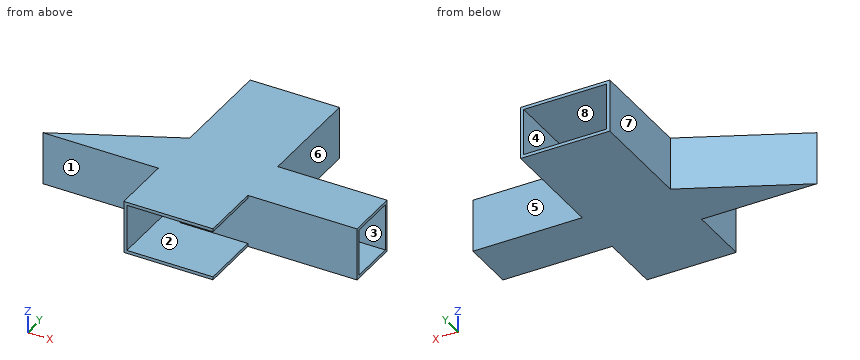
from build123d import *

# Parameters (mm, degrees)
ESQUISSE1_W             = 145
ESQUISSE1_H             = 86
ESQUISSE1_W_2           = 135
ESQUISSE1_H_2           = 76
BOSS_EXTRU_1_DEPTH      = 258
ESQUISSE2_W             = 145
ESQUISSE2_H             = 86
BOSS_EXTRU_2_DEPTH      = 5
ESQUISSE3_W             = 30
ESQUISSE3_H             = 76
ENL_V_MAT_EXTRU_1_DEPTH = 5
ESQUISSE5_W             = 5
ESQUISSE5_H             = 86
BOSS_EXTRU_3_DEPTH      = 100
BOSS_EXTRU_6_DEPTH      = 86
ESQUISSE10_W            = 86
ESQUISSE10_H            = 86
ESQUISSE10_W_2          = 76
ESQUISSE10_H_2          = 76
BOSS_EXTRU_7_DEPTH      = 177.5
ESQUISSE11_W            = 76
ESQUISSE11_H            = 76
ENL_V_MAT_EXTRU_2_DEPTH = 10
ESQUISSE12_W            = 140
ESQUISSE12_H            = 5
BOSS_EXTRU_8_DEPTH      = 100


with BuildPart() as part:
    # Esquisse1 → Boss.-Extru.1 (new body)
    with BuildSketch(Plane(origin=(0, 0, 0), x_dir=(1, 0, 0), z_dir=(0, 1, 0))):
        with Locations((34.799005462, -27.04875873)):
            Rectangle(ESQUISSE1_W, ESQUISSE1_H)
        with Locations((34.799005462, -27.04875873)):
            Rectangle(ESQUISSE1_W_2, ESQUISSE1_H_2, mode=Mode.SUBTRACT)
    extrude(amount=BOSS_EXTRU_1_DEPTH)

    # Esquisse2 → Boss.-Extru.2 (add)
    with BuildSketch(Plane.XZ):
        with Locations((34.799005462, 27.04875873)):
            Rectangle(ESQUISSE2_W, ESQUISSE2_H)
    extrude(amount=BOSS_EXTRU_2_DEPTH)

    # Esquisse3 → Enlèv. mat.-Extru.1 (cut)
    with BuildSketch(Plane.XZ.offset(5)):
        with Locations((-17.700994538, 27.04875873)):
            Rectangle(ESQUISSE3_W, ESQUISSE3_H)
    extrude(amount=-ENL_V_MAT_EXTRU_1_DEPTH, mode=Mode.SUBTRACT)

    # Esquisse5 → Boss.-Extru.3 (add)
    with BuildSketch(Plane.XZ.offset(5)):
        with Locations((-35.200994538, 27.04875873)):
            Rectangle(ESQUISSE5_W, ESQUISSE5_H)
    extrude(amount=BOSS_EXTRU_3_DEPTH)

    # Esquisse9 → Boss.-Extru.6 (add)
    with BuildSketch(Plane.XY.offset(70.04875873)):
        Polygon((-37.700994538, -5.700514768), (-37.700994538, 84.299485232), (-225.200994538, -5.700514768), align=None)
    extrude(amount=-BOSS_EXTRU_6_DEPTH)

    # Esquisse10 → Boss.-Extru.7 (add)
    with BuildSketch(Plane(origin=(107.299005462, 0, 0), x_dir=(0, 0, -1), z_dir=(1, 0, 0))):
        with Locations((-27.04875873, 38)):
            Rectangle(ESQUISSE10_W, ESQUISSE10_H)
        with Locations((-27.04875873, 38)):
            Rectangle(ESQUISSE10_W_2, ESQUISSE10_H_2, mode=Mode.SUBTRACT)
    extrude(amount=BOSS_EXTRU_7_DEPTH)

    # Esquisse11 → Enlèv. mat.-Extru.2 (cut)
    with BuildSketch(Plane(origin=(107.299005462, 0, 0), x_dir=(0, 0, -1), z_dir=(1, 0, 0))):
        with Locations((-27.04875873, 38)):
            Rectangle(ESQUISSE11_W, ESQUISSE11_H)
    extrude(amount=-ENL_V_MAT_EXTRU_2_DEPTH, mode=Mode.SUBTRACT)

    # Esquisse12 → Boss.-Extru.8 (add)
    with BuildSketch(Plane.XZ.offset(5)):
        with Locations((37.299005462, 67.54875873)):
            Rectangle(ESQUISSE12_W, ESQUISSE12_H)
        with Locations((37.299005462, -13.45124127)):
            Rectangle(ESQUISSE12_W, ESQUISSE12_H)
    extrude(amount=BOSS_EXTRU_8_DEPTH)


solid = part.part
Verification items for the finished model (mm, model axes). Face numbers are marked on the shaded views. A direction names the side the tool comes from. Give positions to 0.01 mm unless a question says otherwise; leave off trailing zeros. Loops run counter-clockwise (first coordinate to the right, second up) from the corner with the lowest first, then second, coordinate; pieces in that order, holes last.
1) Thickness scan on line 1 along X through (y, z) = (158.5, 45); line 2 along Z through (x, y) = (-25.5, 102.5); line 3 along Y through (x, z) = (260, 45.5). Record the ranges inside material, lowest first.
2) Depth check by flat-ended pin: pin 1 Ø4 at (y, z) = (-49.5, 45) entering from -X; pin 2 Ø6 at (x, z) = (72, 46) entering from +Y; pin 3 Ø1.5 at (y, z) = (-47.5, -13) entering from +X. Enter the tip coordinate at first touch or a pass-through.
3) Sectioned sample at C-C, the plane y = -72.5. Enter the section's corners in (x, z).
4) Sectioned sample at B-B, the plane z = 5. Enter the section's corners in (x, y), then the cut area to 3 significant figures.
5) Sectioned sample at A-A, the plane x = 133. Enter the section's corners in (y, z), then the cut area to 3 significant figures.
6) Draft check along X on the marked faces 6, 7 and 8. Enter one of: pulls with the +X half, pulls with the -X half, needs draft (parallel to the pull), parting line crosses it, or undercut.
7) Set-up check for the marked faces 1, 2, 3, 4 and 5: record each of +Z, -Z, +X, -X, +Y, -Y from which the full face is reachable in a straight line by a thin tool's end or side.
8) Sectioned sample at D-D, the plane x = 59. Enter the section's corners in (y, z), then the cut area to 3 significant figures.
Answers:
1. line 1: x = -37.7 to -32.7, 102.3 to 107.3
1. line 2: z = -15.95 to -10.95, 65.05 to 70.05
1. line 3: y = -5 to 0, 76 to 81
2. pin 1: stops at x = -37.7
2. pin 2: stops at y = 0
2. pin 3: stops at x = 107.3
3. outline: (-37.7, -15.95) - (107.3, -15.95) - (107.3, -10.95) - (-32.7, -10.95) - (-32.7, 65.05) - (107.3, 65.05) - (107.3, 70.05) - (-37.7, 70.05) - close
4. outline: (-225.2, -5.7) - (-37.7, -5.7) - (-37.7, -105) - (-32.7, -105) - (-32.7, 258) - (-37.7, 258) - (-37.7, 84.3) - close; (-2.7, -5) - (284.8, -5) - (284.8, 0) - (-2.7, 0) - close; (102.3, 76) - (284.8, 76) - (284.8, 81) - (107.3, 81) - (107.3, 258) - (102.3, 258) - close
4. area: 13,500 mm2
5. outline: (-5, -15.95) - (81, -15.95) - (81, 70.05) - (-5, 70.05) - close; hole (0, -10.95) - (76, -10.95) - (76, 65.05) - (0, 65.05) - close
5. area: 1,620 mm2
6. face 6: pulls with the +X half
6. face 7: pulls with the -X half
6. face 8: undercut
7. face 1: +Z, -Z, -X, -Y
7. face 2: none
7. face 3: +X
7. face 4: +Y
7. face 5: +Z, -Z, +X, +Y
8. outline: (-105, -15.95) - (258, -15.95) - (258, -10.95) - (0, -10.95) - (0, 65.05) - (258, 65.05) - (258, 70.05) - (-105, 70.05) - (-105, 65.05) - (-5, 65.05) - (-5, -10.95) - (-105, -10.95) - close
8. area: 4,010 mm2
